Geometry: see drawing. Coordinates: mm, zero at the bounding-box minimum. Give positions to 0.01 mm unless a question says otherwise; leave off trailing zeros. Write each loop counter-clockwise with the first axis right and the second up, starting at its lowest first coordinate (ties: lowest second). Pieces come first, ordered by that corner, then holes. Notation, with made-up numbers: (24.5, -3) - (64.5, -3) arc R27 ccw to (64.5, 19) - close; hole circle Ø9 at (59, -9). An arc over 180 degrees is marked (long way). One line per question, with ' | ' between items. Start each with the question number.
(1) Ray query, line 1 (X direction, y = 85, z = 19.25); line 2 (Y direction, x = 124.5, z = 5) (1 decimal). Return the intervals inside material, ascending. Write a range as [from, to].
(2) Pin query (flat end, axial travel): pin 1 (6 mm diameter, centred on y = 32.5, z = 24, fed in from -X); pin 2 (12 mm diameter, centred on x = 45.5, z = 15.5, fed in from -Y); pin 3 (2 mm diameter, centred on y = 165, z = 12.5, fed in from -X). Return the tip coordinate at first contact, or that it passes through.
(3) Section B-B, the plane y = 116. Return loops of the section in (x, z) (1 decimal), plus the area to 3 significant figures.
(4) Section C-C, the plane x = 147.5. Return loops of the section in (y, z).
(5) Section A-A, the plane z = 16.75. Return loops of the section in (x, y).
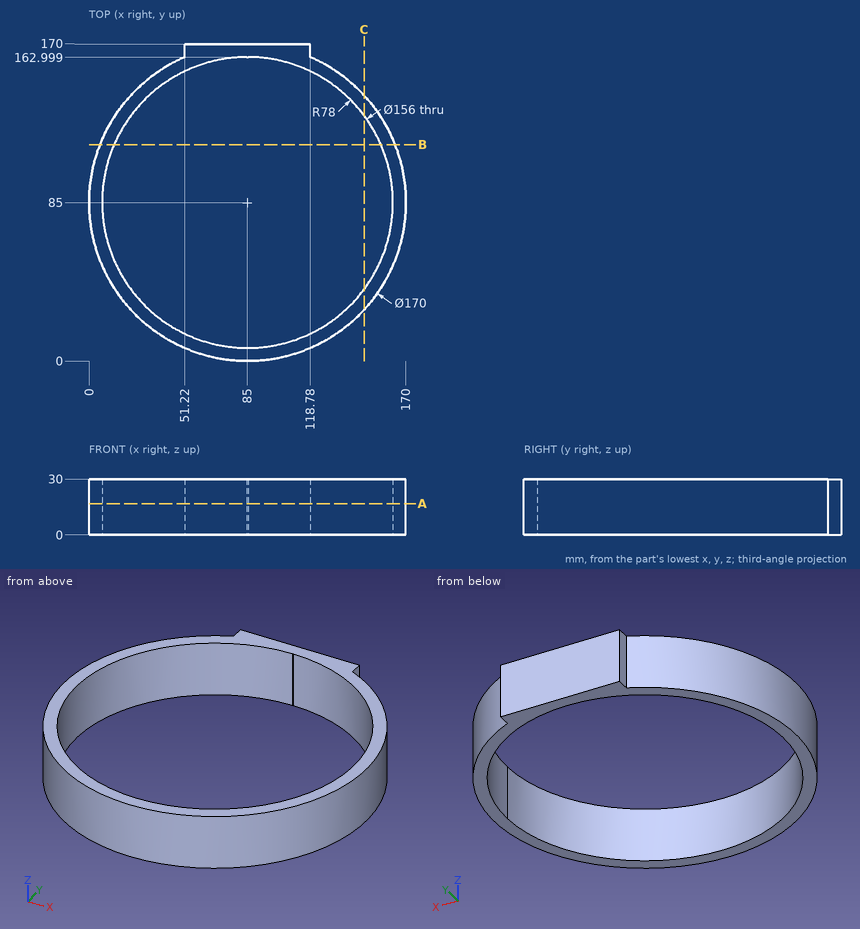
Check sheet entries:
1) line 1: [0, 7], [163, 170] | line 2: [9.7, 17.7], [152.3, 160.3]
2) pin 1: x = 15.9 | pin 2: y = 6.88 | pin 3: x = 51.22
3) outline: (5.9, 0) - (13.4, 0) - (13.4, 30) - (5.9, 30) - close; (156.6, 0) - (164.1, 0) - (164.1, 30) - (156.6, 30) - close | area: 454 mm²
4) outline: (27.39, 0) - (38.33, 0) - (38.33, 30) - (27.39, 30) - close; (131.67, 0) - (142.61, 0) - (142.61, 30) - (131.67, 30) - close
5) outline: (51.22, 163) arc R85 ccw (long way) to (118.78, 163) - (118.78, 170) - (51.22, 170) - close; hole (84.7, 163) arc R78 ccw (long way) to (85.3, 163) - close
